Geometry: final body of the model. Coordinates: model frame, mm. A direction names the side the tool comes from. Round coordinates to 2 decimals unless told otherwise and drop trailing zeros. Order: outer loops, then holes, each group sorted by start corner. A loop starts at its lowest first (then second) coordinate and runs counter-clockwise, first axis right, second up. Notation, with made-up numbers: M 79,81.25 L 87,81.25 A26 ccw 87,117.25 Z; hole C -27,45 d2. An arc over 180 degrees is marked long. Put each result on its own line as item: value. Start each with the question number.
1) First-contact query: P1, Ø5, axis at x = -28.5, y = 9.5, coming from the +Z side; P2, Ø3, axis at x = 1.5, z = -20.5, coming from the -Y side; P3, Ø3, axis at x = 0, z = -22.5, coming from the -Y side. Flat tips, straight axial feed; report the tip coordinate or a pass-through.
2) Section C-C, the plane x = 30. Return loops of the section in (y, z), then the cut area to 3 significant figures.
3) Section B-B, the plane z = 6. Return loops of the section in (x, y), then the cut area to 3 significant figures.
4) Access query for faces 4 (the flat face through (-1, 15, -25)), 5 (the flat face through (25.45, 10.81, 22.04)), 6 (the flat face through (0, 4, -18)). Directions: +Z, -Z, +X, -X, +Y, -Y. A direction counts if a zero-diameter tool reaches every point of the face in a straight line with its end or side. Return the directions, or none.
5) Draft query along Y for faces 1 (the flat face through (1, 0, 0)), 2 (the flat face through (30, 3, 22)), 3 (the flat face through (1, 8, 25)). Return one class per face: pulls with the +Y half, pulls with the -Y half, needs draft (parallel to the pull), parting line crosses it, or undercut.
6) Section A-A, the plane x = -30. Return loops of the section in (y, z), then the cut area to 3 significant figures.
7) Section D-D, the plane x = 0. Return loops of the section in (y, z).
8) Material intervals for probe 1 along X at (y, z) = (8, -7); probe 2 along Y at (x, z) = (-30, 8.5); probe 3 along X at (y, z) = (5.75, 12), sorted ascending. Write a range as [from, to].
Autodesk Inventor part; units mm, degrees
ref_plane "YZ Plane" through (0, 0, 0) normal (1, 0, 0) x (0, 1, 0)
ref_plane "XZ Plane" through (0, 0, 0) normal (0, 1, 0) x (-1, 0, 0)
ref_plane "XY Plane" through (0, 0, 0) normal (0, 0, 1) x (1, 0, 0)
sketch "Schizzo1" plane through (0, 0, 0) normal (0, 1, 0) x (-1, 0, 0)
  line L0 (50, -25) -> (-50, -25)
  line L1 (-50, -25) -> (-50, 25)
  line L2 (-50, 25) -> (50, 25)
  line L3 (50, 25) -> (50, -25)
  line L4 (50, -25) -> (-50, 25) construction
  line L5 (-50, -25) -> (50, 25) construction
  point P0 (0, 0)
  point P1 (0, 0)
  point P2 (0, 0)
  dimension "d0" = 50
  dimension "d9" = 100
extrude "Estrusione1" add sketch "Schizzo1" along normal blind 16
sketch "Schizzo2" plane through (0, 0, 0) normal (0, -1, 0) x (1, 0, 0)
  circle A0 centre (0, -25) radius 9.5
  line L0 (50, -25) -> (-50, -25)
  point P0 (0, 0)
  dimension "d3" = 19
extrude "Estrusione2" cut sketch "Schizzo2" against normal blind 4
sketch "Schizzo3" plane through (0, 4, 0) normal (0, -1, 0) x (1, 0, 0)
  circle A0 centre (0, -25) radius 6
  line L0 (9.5, -25) -> (-9.5, -25)
  point P0 (0, 0)
  dimension "d6" = 12
extrude "Estrusione3" cut sketch "Schizzo3" against normal blind 10
sketch "Schizzo4" plane through (-50, 0, 25) normal (0, 0, 1) x (1, 0, 0)
  line L0 (50, 0) -> (50, 8)
  line L1 (50, 0) -> (58, 0) construction
  line L2 (50, 8) -> (20, 8)
  line L3 (50, 8) -> (80, 8)
  line L4 (50, 8) -> (80, 8) construction
  dimension "d10" = 8
  dimension "d11" = 90
  dimension "d12" = 30
  dimension "d13" = 90
  dimension "d14" = 30
  dimension "d15" = 0
hole "Foro1" at (30, 8, 25) at (-30, 8, 25) direction (0, 0, -1) diameter 6.6 end through all
sketch "Schizzo5" plane through (-50, 0, 25) normal (0, 0, 1) x (1, 0, 0)
  circle A0 centre (80, 8) radius 3.3
  circle A1 centre (80, 8) radius 5
  circle A2 centre (20, 8.2293) radius 5
  line L0 (17.1132, 3.2293) -> (14.2265, 8.2293)
  line L1 (14.2265, 8.2293) -> (17.1132, 13.2293)
  line L2 (17.1132, 13.2293) -> (22.8868, 13.2293)
  line L3 (22.8868, 13.2293) -> (25.7735, 8.2293)
  line L4 (25.7735, 8.2293) -> (22.8868, 3.2293)
  line L5 (22.8868, 3.2293) -> (17.1132, 3.2293)
  line L6 (76.9809, 3) -> (73.9618, 8.2293)
  line L7 (73.9618, 8.2293) -> (76.9809, 13.4586)
  line L8 (76.9809, 13.4586) -> (83.0191, 13.4586)
  line L9 (83.0191, 13.4586) -> (86.0382, 8.2293)
  line L10 (86.0382, 8.2293) -> (83.0191, 3)
  line L11 (83.0191, 3) -> (76.9809, 3)
  point P0 (50, 0)
  point P1 (20, 3.2293)
  point P2 (80, 8.2293)
  point P3 (80, 3)
  dimension "d24" = 10
  dimension "d25" = 10
extrude "Estrusione4" cut sketch "Schizzo5" against normal blind 6 contours A0 | A1 | L11 L6 L7 L8 L9 L10 | A2 | A2 L3 L4 | A2 L2 L3 | L4 L5 A2 | A2 L1 L2 | L5 L0 A2 | A2 L0 L1
properties part number "14_base_avanti"
Result sheet:
1. P1: stops at z = 19
1. P2: stops at y = 4
1. P3: stops at y = 14
2. outline: M 0,-25 L 4.7,-25 L 4.7,19 L 3,19 L 3,25 L 0,25 Z; M 11.3,-25 L 16,-25 L 16,25 L 13.46,25 L 13.46,19 L 11.3,19 Z
2. area: 447 mm2
3. outline: M -50,0 L 50,0 L 50,16 L -50,16 Z; hole C -30,8 d6.6; hole C 30,8 d6.6
3. area: 1,530 mm2
4. face 4: -Z, +X, -X, +Y, -Y
4. face 5: +Z
4. face 6: -Z, -Y
5. face 1: pulls with the -Y half
5. face 2: undercut
5. face 3: needs draft
6. outline: M 0,-25 L 4.7,-25 L 4.7,19 L 3.23,19 L 3.23,25 L 0,25 Z; M 11.3,-25 L 16,-25 L 16,25 L 13.23,25 L 13.23,19 L 11.3,19 Z
6. area: 450 mm2
7. outline: M 0,-15.5 L 4,-15.5 L 4,-19 L 14,-19 L 14,-25 L 16,-25 L 16,25 L 0,25 Z
8. probe 1: x = [-50, -33.3], [-26.7, 26.7], [33.3, 50]
8. probe 2: y = [0, 4.7], [11.3, 16]
8. probe 3: x = [-50, -32.41], [-27.59, 27.59], [32.41, 50]
